```python
from build123d import *

# Parameters (mm, degrees)
SKETCH_1_R                = 37.5
EXTRUDE_1_DEPTH           = 24
SKETCH_3_R                = 15
EXTRUDE_2_DEPTH           = 19
HOLE_WIZARD_6_0_6_1_D     = 6
HOLE_WIZARD_6_0_6_1_DEPTH = 15
HOLE_WIZARD_6_0_6_1_TIP   = 1.802581857
FILLET_1_R                = 12
HOLE_WIZARD_M6_2_D        = 5
HOLE_WIZARD_M6_2_DEPTH    = 15
HOLE_WIZARD_M6_2_TIP      = 1.502151548


with BuildPart() as part:
    # 草图1 → 凸台-拉伸1 (new body)
    with BuildSketch(Plane(origin=(0, 0, 0), x_dir=(1, 0, 0), z_dir=(0, 1, 0))):
        with Locations(Location((0, 0, 0), (0, 0, 270))):
            Circle(SKETCH_1_R)
    extrude(amount=EXTRUDE_1_DEPTH)

    # 草图3 → 凸台-拉伸2 (add)
    with BuildSketch(Plane(origin=(0, 24, 0), x_dir=(1, 0, 0), z_dir=(0, 1, 0))):
        with Locations(Location((0, 0, 0), (0, 0, 270))):
            Circle(SKETCH_3_R)
    extrude(amount=EXTRUDE_2_DEPTH)

    # Ø6.0 (6) 直径孔1
    with Locations(Plane(origin=(0, 43, 0), x_dir=(1, 0, 0), z_dir=(0, 1, 0))):
        with Locations((0, 0)):
            Hole(HOLE_WIZARD_6_0_6_1_D / 2, depth=HOLE_WIZARD_6_0_6_1_DEPTH)
            with Locations((0, 0, -(HOLE_WIZARD_6_0_6_1_DEPTH + HOLE_WIZARD_6_0_6_1_TIP / 2))):  # 118° drill point
                Cone(0, HOLE_WIZARD_6_0_6_1_D / 2, HOLE_WIZARD_6_0_6_1_TIP, mode=Mode.SUBTRACT)

    # 圆角1
    fillet_1_edges = [part.edges().sort_by_distance(p)[0] for p in [
        (0, 0, -37.5),
        (0, 24, -37.5),
    ]]
    fillet(fillet_1_edges, radius=FILLET_1_R - 0.0001)  # a hair under: the kernel refuses the full size

    # M6 螺纹孔的螺纹孔钻头2
    with Locations(Plane(origin=(-4.612956818, 32.989820413, -14.273073579), x_dir=(-0.951538238599, 0, 0.307530454563), z_dir=(-0.307530454563, 0, -0.951538238599))):
        with Locations((0, 0)):
            Hole(HOLE_WIZARD_M6_2_D / 2, depth=HOLE_WIZARD_M6_2_DEPTH)
            with Locations((0, 0, -(HOLE_WIZARD_M6_2_DEPTH + HOLE_WIZARD_M6_2_TIP / 2))):  # 118° drill point
                Cone(0, HOLE_WIZARD_M6_2_D / 2, HOLE_WIZARD_M6_2_TIP, mode=Mode.SUBTRACT)


solid = part.part
```
Design review of the part built by this model. Coordinates are the model's own, in mm. A direction names the side the tool comes from. Coordinates: 2 decimals unless noted, no trailing zeros. Loops run counter-clockwise (first coordinate to the right, second up) from the corner with the lowest first, then second, coordinate; pieces in that order, holes last. Notation, with made-up numbers: M -22,69.5 L -6,69.5 A38 ccw -6,108.5 Z; hole C -7,44.25 d5. An arc over 180 degrees is marked long. One line per question, with ' | ' between items.
(1) We need section B-B (y = 4). Give the boundary of the cut face in (x, z).
Filled in:
outline: C 0,0 d68.89
(2) Wall thickness on probe 1 along Y at (x, z) = (15.5, 10.5); probe 2 along Z at (x, y) = (33.5, 17); probe 3 along X at (y, z) = (13, -25.5): over which ranges is each line inside the solid? List them lowest first.
Filled in:
probe 1: y = 0 to 24 | probe 2: z = -14.26 to 14.26 | probe 3: x = -27.44 to 27.44
(3) Draft analysis for pull direction X (two halves, no side actions). For faces 3 (the face through (-0.11, 26.51, 0.51)), 4 (the face through (0, 0, 0)), 5 (the face through (0.66, 33.367, -14.985)), state which applies: released by +X, released by -X, zero draft, split by the parting line, or undercut.
Filled in:
face 3: undercut | face 4: zero draft | face 5: split by the parting line
(4) For pin 1 Ø4 at (y, z) = (19, -24.5) entering from +X; pin 2 Ø6 at (y, z) = (23, -17.5) entering from -X; pin 3 Ø1 at (y, z) = (19, -4) entering from -X; pin 4 Ø8 at (x, y) = (27, 30) entering from -Z, all flat-tipped, find the tip position at first contact; note any pin that passes through.
Filled in:
pin 1: stops at x = 27.79 | pin 2: stops at x = -30.09 | pin 3: stops at x = -35.37 | pin 4: passes through
(5) Machinability: for faces 1 (the face through (-11, 24, 11)), 2 (the face through (4, 43, 0)), which of the approach directions +Z, -Z, +X, -X, +Y, -Y give a long, thin tool a straight path to every point of the face, cutting with its end or side? Answer none if there is none.
Filled in:
face 1: +Y | face 2: +Z, -Z, +X, -X, +Y
(6) We need section A-A (y = 20.5). Give the boundary of the cut face in (x, z), and give its area (3 significant figures).
Filled in:
outline: C 0,0 d67.94 | area: 3,630 mm^2
